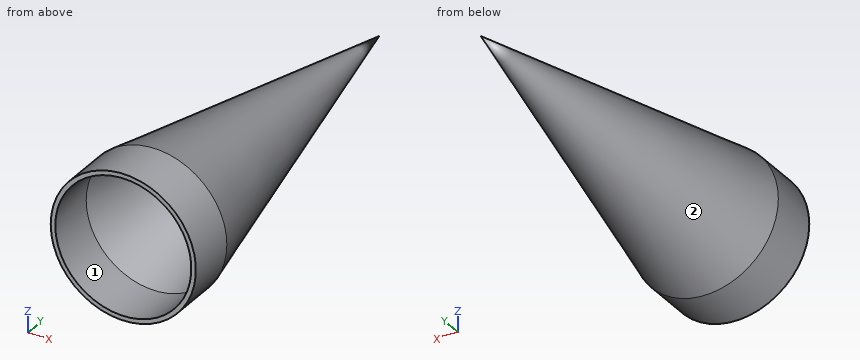
Autodesk Inventor part; units mm, degrees
sketch "Эскиз1" plane through (0, 0, 0) normal (0, 1, 0) x (-1, 0, 0)
  circle A0 centre (0, 0) radius 15
  circle A1 centre (0, 0) radius 16
  dimension "d0" = 30
  dimension "d1" = 32
extrude "Выдавливание1" add sketch "Эскиз1" along normal blind 11
ref_plane "РабПлоскость1" through (0, 91, 0) normal (0, 1, 0) x (1, 0, 0)
sketch "Эскиз3" plane through (0, 91, 0) normal (0, 1, 0) x (1, 0, 0)
  point P0 (0, 0)
  point P1 (0, 0)
  point P2 (0, 0)
sketch "Эскиз4" plane through (0, 11, 0) normal (0, 1, 0) x (1, 0, 0)
  circle A0 centre (0, 0) radius 16
sketch "Эскиз6" plane through (0, 0, 0) normal (0, 0, 1) x (1, 0, 0)
  line L0 (0, 91) -> (16, 11)
  line L1 (0, 111.2721) -> (0, 58.6292)
  line L2 (16, 11) -> (0, 11)
  line L3 (16, 11) -> (-16, 11)
  line L4 (0, 91) -> (0, 11)
  point P0 (0, 0)
  dimension "d10" = 16
  dimension "d11" = 3.9757
  dimension "d12" = 6.3484
revolve "Вращение1" add sketch "Эскиз6" angle 360 about axis through (0, 111.2721, 0) along (0, -1, 0)
sketch "Эскиз7" plane through (0, 0, 0) normal (0, 0, 1) x (1, 0, 0)
  line L0 (15, 11) -> (0, 86)
  line L1 (0, 91) -> (16, 11)
  line L2 (0, 109.2) -> (0, -18.2)
  line L3 (0, 86) -> (0, 11)
  line L4 (-15, 11) -> (15, 11)
  line L5 (0, 11) -> (15, 11)
  point P0 (0, 0)
revolve "Вращение2" cut sketch "Эскиз7" angle 360 about axis through (0, 86, 0) along (0, -1, 0)
properties part number "Головной обтекатель"
Source: CAD feature listing. Evaluate the final solid. Frame: model axes, mm. Face numbers are marked on the shaded views. Round coordinates to 2 decimals unless told otherwise and drop trailing zeros. Loops run counter-clockwise (first coordinate to the right, second up) from the corner with the lowest first, then second, coordinate; pieces in that order, holes last. Notation, with made-up numbers: M 46.25,-15.75 L 69.25,-15.75 A30 cw 69.25,22.25 Z; hole C -22.75,68.5 d1. An arc over 180 degrees is marked long. Return JSON: item names as keys, results as strings. Group by question number.
1. Section query B-B on y = 81. Output: boundary loops of the cut face in (x, z).
2. Material intervals for line 1 along X through (y, z) = (5.25, 0); line 2 along Z through (x, y) = (-2, 14.5), sorted ascending. Write a range as from..to.
3. Pin query (flat end, axial travel): pin 1 (12 mm diameter, centred on x = 7, y = 45.5, fed in from -Z); pin 2 (2 mm diameter, centred on x = -4, y = 69.5, fed in from -Z); pin 3 (8 mm diameter, centred on y = 61, z = 5.5, fed in from +X); pin 4 (10 mm diameter, centred on x = -8.5, z = 6.5, fed in from -Y). Return the tip coordinate at first contact, or that it passes through.
4. Section query A-A on y = 35. Output: boundary loops of the cut face in (x, z), and give its area (3 significant figures).
5. Mould query, pull axis X, two halves, no side actions, for the marked faces 1 and 2. Classes: released by +X, released by -X, zero draft, split by the parting line, or undercut.
Checks:
{
 "1": {"outline": "C 0,0 d4; hole C 0,0 d2"},
 "2": {"line 1": "x = -16..-15, 15..16", "line 2": "z = -15.17..-14.16, 14.16..15.17"},
 "3": {"pin 1": "stops at z = -9.57", "pin 2": "stops at z = -3.12", "pin 3": "stops at x = 6.07", "pin 4": "stops at y = 0"},
 "4": {"outline": "C 0,0 d22.4; hole C 0,0 d20.4", "area": "67.2 mm²"},
 "5": {"face 1": "undercut", "face 2": "split by the parting line"}
}
